```python
from build123d import *

# Parameters (mm, degrees)
F0_W     = 24
F0_H     = 24
F1_DEPTH = 8
F2_R     = 4
F3_W     = 6
F3_H     = 6
F4_DEPTH = 4
F5_R     = 3.75
F6_DEPTH = 18


with BuildPart() as f1:
    # F0 (on Top) → F1 (new body)
    with BuildSketch(Plane.XY):
        Rectangle(F0_W, F0_H)
    extrude(amount=F1_DEPTH)

    # F2
    f2_edges = [f1.edges().sort_by_distance(p)[0] for p in [
        (0, -12, 0),
        (12, 0, 0),
        (0, 12, 0),
        (-12, 0, 0),
        (12, -12, 4),
        (-12, -12, 4),
        (-12, 12, 4),
        (12, 12, 4),
    ]]
    fillet(f2_edges, radius=F2_R)

    # F3 (on face) → F4 (cut)
    with BuildSketch(Plane.XY.offset(8)):
        with Locations((5, 5)):
            Rectangle(F3_W, F3_H)
        with Locations((-5, 5)):
            Rectangle(F3_W, F3_H)
        with Locations((5, -5)):
            Rectangle(F3_W, F3_H)
        with Locations((-5, -5)):
            Rectangle(F3_W, F3_H)
    extrude(amount=-F4_DEPTH, mode=Mode.SUBTRACT)

    # F5 (on face) → F6 (join)
    with BuildSketch(Plane.XY.offset(4)):
        Circle(F5_R)
    extrude(amount=F6_DEPTH)


solid = f1.part
```
Part model, mm, in its own coordinate system. A direction names the side the tool comes from. Give positions to 0.01 mm unless a question says otherwise; leave off trailing zeros. Write each loop counter-clockwise with the first axis right and the second up, starting at its lowest first coordinate (ties: lowest second). Pieces come first, ordered by that corner, then holes. Notation, with made-up numbers: (-11, -1) -> (18, -1) arc R14 ccw to (18, 8) -> close; hole circle Ø11 at (41, -38). An arc over 180 degrees is marked (long way). Put each result on its own line as item: value. Start each with the question number.
Item 1: Cut at B-B (x = 0). List the corners of the cut face in (y, z).
Item 2: Which spindle directions (+Z, -Z, +X, -X, +Y, -Y) get a long thin tool onto all of the face, cutting with end or side? Do faces 1 (the face through (0.112, -10.859, 1.203)), 2 (the face through (-6, 2, 6)). Say none if no direction does.
Item 3: Wall check: L1, parallel to Y at x = 3.75, z = 4.75; L2, parallel to Y at x = 2.75, z = 7; L3, parallel to Z at x = -4.75, y = 4. Give the ranges that are in metal, low to high. Write a range as [from, to].
Item 4: Cut at D-D (x = -4.5). List the corners of the cut face in (y, z).
Item 5: Pull direction Y, two halves, no side cores. Call faces 3 (the face through (0, 12, 6)), 4 (the face through (12, 0, 6)), 5 (the face through (8, 5, 6)): pulls with the +Y half, pulls with the -Y half, needs draft (parallel to the pull), parting line crosses it, or undercut.
Item 6: Pin check, flat tips, straight feed: pin 1 Ø12 at (y, z) = (8, 12) entering from -X; pin 2 Ø5 at (x, y) = (-5.5, -4) entering from +Z; pin 3 Ø4 at (y, z) = (1.5, 16.5) entering from -X; pin 4 Ø4 at (x, z) = (3.5, 12.5) entering from -Y. Stop position of each tip, or through.
Item 7: Cut at A-A (z = 6.75). List the corners of the cut face in (x, y), then the cut area to 3 significant figures.
Answer list:
1. outline: (-12, 4) arc R4 ccw to (-8, 0) -> (8, 0) arc R4 ccw to (12, 4) -> (12, 8) -> (3.75, 8) -> (3.75, 22) -> (-3.75, 22) -> (-3.75, 8) -> (-12, 8) -> close
2. face 1: -Z, +X, -X, -Y
2. face 2: +Z
3. L1: y = [-12, -8], [-2, 2], [8, 12]
3. L2: y = [-12, -8], [-2.55, 2.55], [8, 12]
3. L3: z = [0, 4]
4. outline: (-12, 4) arc R4 ccw to (-8, 0) -> (8, 0) arc R4 ccw to (12, 4) -> (12, 8) -> (8, 8) -> (8, 4) -> (2, 4) -> (2, 8) -> (-2, 8) -> (-2, 4) -> (-8, 4) -> (-8, 8) -> (-12, 8) -> close
5. face 3: pulls with the +Y half
5. face 4: needs draft
5. face 5: undercut
6. pin 1: stops at x = -12
6. pin 2: stops at z = 8
6. pin 3: stops at x = -3.75
6. pin 4: stops at y = -3.44
7. outline: (-12, -8) arc R4 ccw to (-8, -12) -> (8, -12) arc R4 ccw to (12, -8) -> (12, 8) arc R4 ccw to (8, 12) -> (-8, 12) arc R4 ccw to (-12, 8) -> close; hole (-8, -8) -> (-2, -8) -> (-2, -3.17) arc R3.75 cw to (-3.17, -2) -> (-8, -2) -> close; hole (-8, 2) -> (-3.17, 2) arc R3.75 cw to (-2, 3.17) -> (-2, 8) -> (-8, 8) -> close; hole (2, -8) -> (8, -8) -> (8, -2) -> (3.17, -2) arc R3.75 cw to (2, -3.17) -> close; hole (2, 3.17) arc R3.75 cw to (3.17, 2) -> (8, 2) -> (8, 8) -> (2, 8) -> close
7. area: 421 mm2
